Can you work these out from the model? Positions are in its coordinate system, mm. Face numbers are marked on the shaded views. Coordinates: 2 decimals unless noted, no trailing zeros. Order: outer loops, then holes, each group sorted by start corner. A loop starts at its lowest first (then second) coordinate and runs counter-clockwise, first axis right, second up. Notation, with made-up numbers: (-3, 58.5) - (40, 58.5) arc R7 cw to (40, 62.5) - close; hole circle Ø10 at (25.25, -35.75). An arc over 180 degrees is marked (long way). Return JSON: item names as keys, results as strings. Group by question number.
1) If I drill on line 1 along Z through (x, y) = (0, -8.75); line 2 along X through (y, z) = (-9.25, 1.75); line 3 along Z through (x, y) = (-3, -8.5), over which ranges is the centre line in solid material (lowest first)?
2) If we mould it in two halves opening along X, with no side actions, what happens to the marked faces 1, 2 and 3? For each: pulls with the +X half, pulls with the -X half, needs draft (parallel to the pull), parting line crosses it, or undercut.
3) Imagine slicing it at A-A (y = -2.25). Write out the boundary of the cut face in (x, z).
4) For pin 1 Ø2 at (x, z) = (8, -3) entering from -Y; pin 2 Ø5 at (y, z) = (-7.5, -5) entering from -X; pin 3 Ø12 at (x, z) = (-5, 4) entering from -Y, each with a flat end and sliding along its axis, tell me the tip position at first contact or that it passes through.
5) Imagine slicing it at B-B (y = -11.5). Write out the boundary of the cut face in (x, z), and give its area (3 significant figures).
```python
from build123d import *

# Parameters (mm, degrees)
M4X0_7_TAPPED_HOLE1_D           = 3.3
M4X0_7_TAPPED_HOLE1_DEPTH       = 6.508579979
M4X0_7_TAPPED_HOLE1_CSINK_D     = 4.05
M4X0_7_TAPPED_HOLE1_CSINK_ANGLE = 90
M4X0_7_TAPPED_HOLE1_TIP         = 0.991420021


with BuildPart() as part:
    # Sketch1 → Revolve1 (revolve)
    with BuildSketch(Plane.XY, mode=Mode.PRIVATE) as revolve1_sk:
        with BuildLine():
            Line((0, 0), (-11, 0))
            Line((-11, 0), (-11, -4))
            Line((-11, -4), (-5.25, -10))
            Line((-5.25, -10), (-4.5, -10))
            Line((-4.5, -10), (-4.5, -8.3))
            Line((-4.5, -8.3), (-4.2, -8.3))
            ThreePointArc((-4.2, -8.3), (-2.969848481, -11.269848481), (0, -12.5))
            Line((0, -12.5), (0, 0))
        make_face()
    revolve(revolve1_sk.sketch.rotate(Axis((0, -12.5, 0), (0, 1, 0)), 180), axis=Axis((0, -12.5, 0), (0, 1, 0)))

    # M4x0.7 Tapped Hole1
    with Locations(Plane(origin=(0, 0, 0), x_dir=(1, 0, 0), z_dir=(0, 1, 0))):
        with Locations((0, 0)):
            CounterSinkHole(M4X0_7_TAPPED_HOLE1_D / 2, M4X0_7_TAPPED_HOLE1_CSINK_D / 2, depth=M4X0_7_TAPPED_HOLE1_DEPTH, counter_sink_angle=M4X0_7_TAPPED_HOLE1_CSINK_ANGLE)
            with Locations((0, 0, -(M4X0_7_TAPPED_HOLE1_DEPTH + M4X0_7_TAPPED_HOLE1_TIP / 2))):  # 118° drill point
                Cone(0, M4X0_7_TAPPED_HOLE1_D / 2, M4X0_7_TAPPED_HOLE1_TIP, mode=Mode.SUBTRACT)


solid = part.part
```
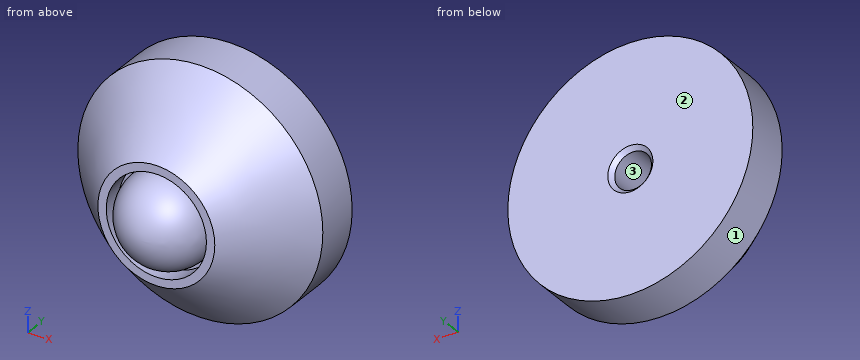
Calculated:
{
 "1": {"line 1": "-6.45 to -4.5, -4.18 to 4.18, 4.5 to 6.45", "line 2": "-5.71 to -4.15, -3.7 to 3.7, 4.15 to 5.71", "line 3": "-5.98 to -3.35, -2.93 to 2.93, 3.35 to 5.98"},
 "2": {"face 1": "parting line crosses it", "face 2": "needs draft", "face 3": "undercut"},
 "3": {"outline": "circle Ø22 at (0, 0); hole circle Ø3.3 at (0, 0)"},
 "4": {"pin 1": "y = -7.61", "pin 2": "x = -8.99", "pin 3": "y = -12.48"},
 "5": {"outline": "circle Ø5.44 at (0, 0)", "area": "23.2 mm2"}
}
